```python
from build123d import *

# Parameters (mm, degrees)
EXTRUDE_1_DEPTH          = 80
CUT_EXTRUDE_1_DEPTH      = 80
CUT_EXTRUDE_1_DEPTH_BACK = 80
SKETCH_2_OUTSIDE_W       = 249.571
SKETCH_2_OUTSIDE_H       = 126.166
EXTRUDE_2_DEPTH          = 80
SKETCH_3_R               = 3
SKETCH_3_R_2             = 2.75
CUT_EXTRUDE_2_DEPTH      = 9
CUT_EXTRUDE_3_DEPTH      = 16
CUT_EXTRUDE_3_DEPTH_BACK = 8
SKETCH_4_W               = 130
SKETCH_4_H               = 1.2
CUT_EXTRUDE_4_DEPTH      = 80
CUT_EXTRUDE_4_DEPTH_BACK = 80
SKETCH_6_OUTSIDE_W       = 274.986
SKETCH_6_OUTSIDE_H       = 130.25
CUT_EXTRUDE_5_DEPTH      = 4
CUT_EXTRUDE_5_DEPTH_BACK = 10
SKETCH_7_W               = 148.853321433
SKETCH_7_H               = 1.2
EXTRUDE_START            = 25
EXTRUDE_3_DEPTH          = 30


with BuildPart() as part:
    # Sketch 1 → Extrude 1 (new body)
    with BuildSketch(Plane.XY):
        with BuildLine():
            ThreePointArc((0.955064977, 5.416442642), (50.154483855, -0.584955192), (99.652703645, 1.969615506))
            Line((99.652703645, 1.969615506), (100, 0))
            ThreePointArc((100, 0), (50, -4.374433176), (0, 0))
            Line((0, 0), (-103.404814066, 18.233058655))
            Line((-103.404814066, 18.233058655), (-101.841980467, 27.096328432))
            Line((-101.841980467, 27.096328432), (0.955064977, 5.416442642))
        make_face()
    extrude(amount=EXTRUDE_1_DEPTH)

    # Sketch 2 outside → Cut-Extrude 1 (cut, two sides: drawn at the far end of the back side and taken through both)
    with BuildSketch(Plane(origin=(0, 0, 0), x_dir=(1, 0, 0), z_dir=(0, 1, 0)).offset(-CUT_EXTRUDE_1_DEPTH_BACK)):
        with Locations((-1.7025, -40)):
            Rectangle(SKETCH_2_OUTSIDE_W, SKETCH_2_OUTSIDE_H)
        with BuildLine():
            Line((-81.404814066, -15), (50, -10))
            ThreePointArc((50, -10), (65.598710239, -11.535484205), (80.598631148, -16.082994028))
            ThreePointArc((80.598631148, -16.082994028), (83.701137928, -18.110683802), (85.85203147, -21.129082567))
            ThreePointArc((85.85203147, -21.129082567), (90, -40), (85.85203147, -58.870917433))
            ThreePointArc((85.85203147, -58.870917433), (83.701137928, -61.889316198), (80.598631148, -63.917005972))
            ThreePointArc((80.598631148, -63.917005972), (65.598710239, -68.464515795), (50, -70))
            Line((50, -70), (-81.404814066, -65))
            ThreePointArc((-81.404814066, -65), (-86.503052151, -64.626694449), (-91.492535917, -63.514741053))
            ThreePointArc((-91.492535917, -63.514741053), (-94.787242262, -61.803307698), (-97.230517167, -59.007864662))
            ThreePointArc((-97.230517167, -59.007864662), (-102.404814066, -40), (-97.230517167, -20.992135338))
            ThreePointArc((-97.230517167, -20.992135338), (-94.787242262, -18.196692302), (-91.492535917, -16.485258947))
            ThreePointArc((-91.492535917, -16.485258947), (-86.503052151, -15.373305551), (-81.404814066, -15))
        make_face(mode=Mode.SUBTRACT)
    extrude(amount=CUT_EXTRUDE_1_DEPTH + CUT_EXTRUDE_1_DEPTH_BACK, mode=Mode.SUBTRACT)

    # Sketch 5 → Extrude 2 (add)
    with BuildSketch(Plane.XY):
        with BuildLine():
            Line((0.130982352, -0.692946324), (-41.136860859, 2.924444243))
            ThreePointArc((-41.136860859, 2.924444243), (-60.962244436, 2.718445526), (-80.369357278, -1.337690645))
            ThreePointArc((-80.369357278, -1.337690645), (-107.081623518, -5.831422582), (-134.01223301, -2.919195453))
            Line((-134.01223301, -2.919195453), (-134.739648073, -5.8296709))
            ThreePointArc((-134.739648073, -5.8296709), (-106.993215622, -8.83011964), (-79.471740806, -4.200256744))
            ThreePointArc((-79.471740806, -4.200256744), (-60.638237212, -0.264006371), (-41.398825562, -0.064096286))
            Line((-41.398825562, -0.064096286), (-0.130982352, -3.681486853))
            Line((-0.130982352, -3.681486853), (9.869017648, -4.558050852))
            Line((9.869017648, -4.558050852), (10.130982352, -1.569510322))
            Line((10.130982352, -1.569510322), (0.130982352, -0.692946324))
        make_face()
    extrude(amount=EXTRUDE_2_DEPTH)

    # Sketch 3 → Cut-Extrude 2 (cut)
    with BuildSketch(Plane(origin=(1.134352673, 5.378630886, 0), x_dir=(0.9784760335424555, -0.206360489878813, 0), z_dir=(0.206360489878813, 0.9784760335424555, 0))):
        with Locations(Location((-74.207967172, -40, 0), (0, 0, 180))):
            Circle(SKETCH_3_R)
        with Locations(Location((-74.207967172, -28, 0), (0, 0, 180))):
            Circle(SKETCH_3_R_2)
        with Locations(Location((-63.815662327, -34, 0), (0, 0, 180))):
            Circle(SKETCH_3_R_2)
        with Locations(Location((-63.815662327, -46, 0), (0, 0, 180))):
            Circle(SKETCH_3_R_2)
        with Locations(Location((-74.207967172, -52, 0), (0, 0, 180))):
            Circle(SKETCH_3_R_2)
        with Locations(Location((-84.600272018, -46, 0), (0, 0, 180))):
            Circle(SKETCH_3_R_2)
        with Locations(Location((-84.600272018, -34, 0), (0, 0, 180))):
            Circle(SKETCH_3_R_2)
    extrude(amount=-CUT_EXTRUDE_2_DEPTH, mode=Mode.SUBTRACT)

    # Sketch 4 → Cut-Extrude 3 (cut, two sides: drawn at the far end of the back side and taken through both)
    with BuildSketch(Plane(origin=(0, 0, 0), x_dir=(1, 0, 0), z_dir=(0, 1, 0)).offset(-CUT_EXTRUDE_3_DEPTH_BACK)):
        with Locations((40, -40)):
            Rectangle(SKETCH_4_W, SKETCH_4_H)
    extrude(amount=CUT_EXTRUDE_3_DEPTH + CUT_EXTRUDE_3_DEPTH_BACK, mode=Mode.SUBTRACT)

    # Sketch 6 outside → Cut-Extrude 4 (cut, two sides: drawn at the far end of the back side and taken through both)
    with BuildSketch(Plane(origin=(0, 0, 0), x_dir=(1, 0, 0), z_dir=(0, 1, 0)).offset(-CUT_EXTRUDE_4_DEPTH_BACK)):
        with Locations((-22.372, -40)):
            Rectangle(SKETCH_6_OUTSIDE_W, SKETCH_6_OUTSIDE_H)
        with BuildLine():
            Line((136.18747393, -6.720535905), (136.18747393, -73.279464095))
            Line((136.18747393, -73.279464095), (-81.404814066, -65))
            ThreePointArc((-81.404814066, -65), (-93.222494497, -63.824675343), (-104.577187887, -60.344747642))
            ThreePointArc((-104.577187887, -60.344747642), (-108.681527165, -57.165161548), (-110.63849353, -52.356247816))
            ThreePointArc((-110.63849353, -52.356247816), (-111.404814066, -40), (-110.63849353, -27.643752184))
            ThreePointArc((-110.63849353, -27.643752184), (-108.681527165, -22.834838452), (-104.577187887, -19.655252358))
            ThreePointArc((-104.577187887, -19.655252358), (-93.222494497, -16.175324657), (-81.404814066, -15))
            Line((-81.404814066, -15), (136.18747393, -6.720535905))
        make_face(mode=Mode.SUBTRACT)
    extrude(amount=CUT_EXTRUDE_4_DEPTH + CUT_EXTRUDE_4_DEPTH_BACK, mode=Mode.SUBTRACT)

    # Sketch 7 → Cut-Extrude 5 (cut, two sides: drawn at the far end of the back side and taken through both)
    with BuildSketch(Plane(origin=(0, 0, 0), x_dir=(1, 0, 0), z_dir=(0, 1, 0)).offset(-CUT_EXTRUDE_5_DEPTH_BACK)):
        with Locations((-99.426660717, -40)):
            Rectangle(SKETCH_7_W, SKETCH_7_H)
    extrude(amount=CUT_EXTRUDE_5_DEPTH + CUT_EXTRUDE_5_DEPTH_BACK, mode=Mode.SUBTRACT)

    # Sketch 8 → Extrude 3 (add)
    with BuildSketch(Plane.XY.offset(EXTRUDE_START)):
        Polygon((-110.63849353, -8.872435364), (65.321019644, -3.966533563), (69.680983926, -3.134969109), (69.680983926, -3.944974028), (-110.63849353, -8.972435364), align=None)
    extrude(amount=EXTRUDE_3_DEPTH)


solid = part.part
```
Verification items for the finished model (mm, model axes). A direction names the side the tool comes from. Give positions to 0.01 mm unless a question says otherwise; leave off trailing zeros. Loops run counter-clockwise (first coordinate to the right, second up) from the corner with the lowest first, then second, coordinate; pieces in that order, holes last.
1. Set-up check for faces 3 (the cylindrical face through (-86.574, 19.56, 15.384)), 4 (the flat face through (-50.486, 8.902, 39.607)), 5 (the cylindrical face through (-102.404, 22.051, 40.279)): record each of +Z, -Z, +X, -X, +Y, -Y from which the full face is reachable in a straight line by a thin tool's end or side.
2. Mould release check, pull along Y, two halves, no side actions. Record for faces 1 (the cylindrical face through (44.67, -0.34, 24.49)), 2 (the cylindrical face through (41.722, -4.255, 24.494)): released by +Y, released by -Y, zero draft, split by the parting line, or undercut.
3. Section check B-B, the plane x = -7. Enter the section's corners in (y, z), then the cut area to 3 significant figures.
4. Section check A-A, the plane x = 47.5. Enter the section's corners in (y, z), then the cut area to 3 significant figures.
5. Thickness scan on line 1 (Z direction, x = -73, y = -1); line 2 (Y direction, x = -83.5, z = 58); line 3 (Z direction, x = 54, y = -2.5). Record the ranges inside material, lowest first.
6. Go/stop test with flat-tipped pins: pin 1 Ø10 at (x, z) = (-57.5, 42.5) entering from +Y; pin 2 Ø12 at (x, z) = (66, 58) entering from +Y; pin 3 Ø21.5 at (x, y) = (21, 2) entering from -Z. Record where each tip stops, or that it passes through.
Geometry says:
1. face 3: -Z, -X, +Y
1. face 4: +Z, -Z
1. face 5: -X, +Y
2. face 1: released by +Y
2. face 2: undercut
3. outline: (-6.08, 25) - (-5.98, 25) - (-5.98, 55) - (-6.08, 55) - close; (-3.08, 12.17) - (-0.07, 12.17) - (-0.07, 39.4) - (-3.08, 39.4) - close; (-3.08, 40.6) - (-0.07, 40.6) - (-0.07, 67.83) - (-3.08, 67.83) - close; (1.23, 12.17) - (7.09, 12.17) - (7.09, 39.4) - (1.23, 39.4) - close; (1.23, 40.6) - (7.09, 40.6) - (7.09, 67.83) - (1.23, 67.83) - close
3. area: 486 mm2
4. outline: (-4.56, 25) - (-4.46, 25) - (-4.46, 55) - (-4.56, 55) - close; (-4.36, 10.1) - (-0.48, 10.1) - (-0.48, 39.4) - (-4.36, 39.4) - close; (-4.36, 40.6) - (-0.48, 40.6) - (-0.48, 69.9) - (-4.36, 69.9) - close
4. area: 231 mm2
5. line 1: z = 14.68 to 39.4, 40.6 to 65.32
5. line 2: y = -5.37 to -2.26, 14.72 to 23.23
5. line 3: z = 10.1 to 39.4, 40.6 to 69.9
6. pin 1: stops at y = 18.8
6. pin 2: stops at y = -0.52
6. pin 3: stops at z = 10.7
